Here's how the part is built. I have some questions about the finished solid (model axes, mm). A direction names the side the tool comes from. Give positions to 0.01 mm unless a question says otherwise; leave off trailing zeros. Write each loop counter-clockwise with the first axis right and the second up, starting at its lowest first coordinate (ties: lowest second). Pieces come first, ordered by that corner, then holes. Notation, with made-up numbers: (-12, 82) -> (27, 82) arc R20 cw to (27, 120) -> close; hole circle Ø10 at (61, 77). An arc over 180 degrees is marked (long way). Use CSV: the item, a comma, the result in double quotes. Start each with the question number.
(1) Suppose I cut it at A-A on y = 0. List the corners of the cut face in (x, z) for me.
(2) If we mould it in two halves opening along Z, with no side actions, what happens to faces 1 (the flat face through (6.35, 3, -1)), 2 (the cylindrical face through (-5.103, 2.45, -3.195)), 3 (the cylindrical face through (0.085, 1.468, -1.915))? For each: pulls with the +Z half, pulls with the -Z half, needs draft (parallel to the pull), parting line crosses it, or undercut.
(3) For pin 1 Ø1.5 at (x, z) = (-1, 1) entering from +Y; pin 2 Ø2 at (x, z) = (-4.5, 4) entering from +Y; pin 3 Ø6 at (x, z) = (-3, 3.5) entering from -Y, each with a flat end and sliding along its axis, tell me the tip position at first contact or that it passes through.
(4) Which directions (+Z, -Z, +X, -X, +Y, -Y) give clear straight access to the entire face, cutting with the end or side of a thin tool? Please do faces 4 (the flat face through (-6.35, 3, 1)), 5 (the cylindrical face through (5.067, 2.45, -3.195)).
(5) I need wall thicknesses on L1, parallel to Y at x = -0.75, z = -1; L2, parallel to Y at x = 2.25, z = 0; L3, parallel to Z at x = 2.5, y = 1. Which ranges of each line are inside material? Lowest first, please. Write a range as [from, to].
(6) Suppose I cut it at D-D on x = -0.5. List the corners of the cut face in (y, z) for me.
(7) Suppose I cut it at C-C on z = 3.75. List the corners of the cut face in (x, y) for me.
from build123d import *

# Parameters (mm, degrees)
CHAMFER1_SIZE = 0.254


with BuildPart() as part:
    # Sketch1 → Revolve1 (revolve)
    with BuildSketch(Plane.XY, mode=Mode.PRIVATE) as revolve1_sk:
        with BuildLine():
            Line((-6.35, 4.0259), (-6.35, 2.413))
            Line((-6.35, 2.413), (6.35, 2.413))
            Line((6.35, 2.413), (6.35, 4.0259))
            Line((6.35, 4.0259), (3.820146489, 4.0259))
            ThreePointArc((3.820146489, 4.0259), (0, 5.5499), (-3.820146489, 4.0259))
            Line((-3.820146489, 4.0259), (-6.35, 4.0259))
        make_face()
    revolve(revolve1_sk.sketch.rotate(Axis((-18.157637283, 0, 0), (1, 0, 0)), 90), axis=Axis((-18.157637283, 0, 0), (1, 0, 0)))

    # Chamfer1
    chamfer1_edges = [part.edges().sort_by_distance(p)[0] for p in [
        (-6.35, 0, -2.413),
        (6.35, 0, -2.413),
    ]]
    chamfer(chamfer1_edges, length=CHAMFER1_SIZE)


solid = part.part
Geometry says:
1,outline,"(-6.35, -4.03) -> (-3.82, -4.03) arc R5.55 ccw to (3.82, -4.03) -> (6.35, -4.03) -> (6.35, -2.67) -> (6.1, -2.41) -> (-6.1, -2.41) -> (-6.35, -2.67) -> close; (-6.35, 2.67) -> (-6.1, 2.41) -> (6.1, 2.41) -> (6.35, 2.67) -> (6.35, 4.03) -> (3.82, 4.03) arc R5.55 ccw to (-3.82, 4.03) -> (-6.35, 4.03) -> close"
2,face 1,"needs draft"
2,face 2,"parting line crosses it"
2,face 3,"undercut"
3,pin 1,"y = 5.51"
3,pin 2,"y = 2.68"
3,pin 3,"y = -5.31"
4,face 4,"+Z, -Z, -X, +Y, -Y"
4,face 5,"+X"
5,L1,"[-5.41, -2.2], [2.2, 5.41]"
5,L2,"[-5.07, -2.41], [2.41, 5.07]"
5,L3,"[-4.85, -2.2], [2.2, 4.85]"
6,outline,"circle Ø11.05 at (0, 0); hole circle Ø4.83 at (0, 0)"
7,outline,"(-6.35, -1.46) -> (-3.82, -1.46) arc R4.09 ccw to (3.82, -1.46) -> (6.35, -1.46) -> (6.35, 1.46) -> (3.82, 1.46) arc R4.09 ccw to (-3.82, 1.46) -> (-6.35, 1.46) -> close"
